Geometry check sheet. Reference: the model listing, model coordinates, mm. Coordinates: 2 decimals unless noted, no trailing zeros. Loops run counter-clockwise (first coordinate to the right, second up) from the corner with the lowest first, then second, coordinate; pieces in that order, holes last. Notation, with made-up numbers: M 69.25,64.25 L 106.25,64.25 A19 ccw 106.25,95.25 Z; hole C 57,-33.5 d8. An arc over 180 degrees is marked long. Use CSV: the item, a comma, the result in double quotes.
```python
from build123d import *

# Parameters (mm, degrees)
SKETCH_1_R      = 2
SKETCH_1_R_2    = 2.05
SKETCH_1_R_3    = 1.25
EXTRUDE_1_DEPTH = 2
FILLET_1_R      = 2
FILLET_3_R      = 9


with BuildPart() as part:
    # 草图1 → 凸台-拉伸1 (new body)
    with BuildSketch(Plane.XY):
        with BuildLine():
            Line((14.659550972, 15.317683161), (14.659550972, 31.317683161))
            Line((14.659550972, 31.317683161), (-4.340449028, 31.317683161))
            Line((-4.340449028, 31.317683161), (-4.340449028, 92.729225893))
            ThreePointArc((-4.340449028, 92.729225893), (-13.340449028, 126.317683161), (-22.340449028, 92.729225893))
            Line((-22.340449028, 92.729225893), (-22.340449028, 69.989347616))
            ThreePointArc((-22.340449028, 69.989347616), (-18.993837092, 68.603135564), (-17.60762504, 65.256523627))
            Line((-17.60762504, 65.256523627), (-30.009910092, 65.256523627))
            Line((-30.009910092, 65.256523627), (-31.902307309, 60.456523627))
            Line((-31.902307309, 60.456523627), (-41.340449028, 60.456523627))
            Line((-41.340449028, 60.456523627), (-41.340449028, 31.317683161))
            Line((-41.340449028, 31.317683161), (-41.340449028, 15.317683161))
            Line((-41.340449028, 15.317683161), (14.659550972, 15.317683161))
        make_face()
        with Locations((-33.340449028, 23.317683161)):
            Circle(SKETCH_1_R, mode=Mode.SUBTRACT)
        with Locations(Location((6.659550972, 23.317683161, 0), (0, 0, 180))):
            Circle(SKETCH_1_R, mode=Mode.SUBTRACT)
        with Locations((-13.340449028, 108.317683161)):
            Circle(SKETCH_1_R, mode=Mode.SUBTRACT)
        with Locations((-13.340449028, 43.317683161)):
            Circle(SKETCH_1_R, mode=Mode.SUBTRACT)
        with Locations((-4.840449028, 116.817683161)):
            Circle(SKETCH_1_R_2, mode=Mode.SUBTRACT)
        with Locations((-31.902307309, 51.317683161)):
            Circle(SKETCH_1_R_3, mode=Mode.SUBTRACT)
        with Locations((-4.840449028, 99.817683161)):
            Circle(SKETCH_1_R_2, mode=Mode.SUBTRACT)
        with Locations((-21.840449028, 99.817683161)):
            Circle(SKETCH_1_R_2, mode=Mode.SUBTRACT)
        with Locations((-21.840449028, 116.817683161)):
            Circle(SKETCH_1_R_2, mode=Mode.SUBTRACT)
        with BuildLine():
            ThreePointArc((-26.536162252, 42.002803279), (-21.278560655, 49.674969847), (-23.973383464, 58.576792381))
            ThreePointArc((-23.973383464, 58.576792381), (-25.73943382, 58.654677802), (-25.817319241, 56.888627446))
            ThreePointArc((-25.817319241, 56.888627446), (-23.749199411, 50.056996199), (-27.784102963, 44.169054414))
            ThreePointArc((-27.784102963, 44.169054414), (-28.243258175, 42.461958491), (-26.536162252, 42.002803279))
        make_face(mode=Mode.SUBTRACT)
    extrude(amount=EXTRUDE_1_DEPTH)

    # 圆角1
    fillet_1_edges = [part.edges().sort_by_distance(p)[0] for p in [
        (-41.340449028, 15.317683161, 1),
        (-30.009910092, 65.256523627, 1),
        (-17.60762504, 65.256523627, 1),
        (-22.340449028, 69.989347616, 1),
        (-22.340449028, 92.729225893, 1),
        (-4.340449028, 92.729225893, 1),
        (-4.340449028, 31.317683161, 1),
        (14.659550972, 31.317683161, 1),
        (14.659550972, 15.317683161, 1),
    ]]
    fillet(fillet_1_edges, radius=FILLET_1_R)

    # 圆角3
    fillet_3_edges = [part.edges().sort_by_distance(p)[0] for p in [
        (-41.340449028, 60.456523627, 1),
    ]]
    fillet(fillet_3_edges, radius=FILLET_3_R)


solid = part.part
```
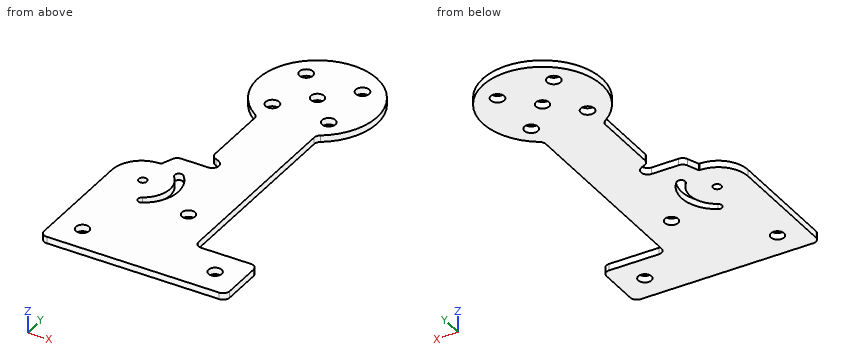
1. Gauge pin test, flat ends, axial feed: P1, Ø3.5, axis at x = 6.66, y = 23.32, coming from the +Z side; P2, Ø1, axis at y = 78, z = 1, coming from the -X side. Record the tip position at first contact, or that the pin passes through.
The answers:
P1,"through"
P2,"x = -22.34"
2. Section check D-D, the plane y = 113.5. Record the cut outline in (x, z).
The answers:
outline,"M -30.58,0 L 3.9,0 L 3.9,2 L -30.58,2 Z"
3. Thickness scan on line 1 (Y direction, x = -32, z = 0.3); line 2 (Y direction, x = -13.5, z = 0.1); line 3 (X direction, y = 101, z = 1.95). Record the ranges inside material, lowest first. Write a range as [from, to].
The answers:
line 1,"[15.32, 21.83], [24.8, 50.07], [52.56, 60.46]"
line 2,"[15.32, 41.32], [45.31, 106.32], [110.31, 126.32]"
line 3,"[-29.79, -23.52], [-20.17, -6.52], [-3.17, 3.1]"
4. Section check C-C, the plane y = 89. Record the cut outline in (x, z), plus the area to 3 significant figures.
The answers:
outline,"M -22.34,0 L -4.34,0 L -4.34,2 L -22.34,2 Z"
area,"36.0 mm^2"
5. Section check A-A, the plane x = 0. Record the cut outline in (y, z), plus the area to 3 significant figures.
The answers:
outline,"M 15.32,0 L 31.32,0 L 31.32,2 L 15.32,2 Z; M 96.23,0 L 120.4,0 L 120.4,2 L 96.23,2 Z"
area,"80.3 mm^2"
6. Section check B-B, the plane z = 0.3. Count the separate pieces of the cut face and the enclosed holes in it, plus the area to 3 significant figures.
The answers:
separate pieces,"1"
enclosed holes,"10"
area,"3,390 mm^2"
